Geometry: final body of the model. Coordinates: model frame, mm. A direction names the side the tool comes from. Give positions to 0.01 mm unless a question says otherwise; leave off trailing zeros. Loops run counter-clockwise (first coordinate to the right, second up) from the corner with the lowest first, then second, coordinate; pieces in that order, holes last. Notation, with made-up numbers: (21, -16.5) - (75, -16.5) arc R13 cw to (75, -2.5) - close; hole circle Ø5 at (-19, 72). An arc over 180 degrees is marked (long way). Answer in a Markdown table with one row per item.
from build123d import *

# Parameters (mm, degrees)
SKETCH1_W           = 406.4
SKETCH1_H           = 215.9
BOSS_EXTRUDE1_DEPTH = 12.7
SKETCH3_W           = 406.4
SKETCH3_H           = 190.5
CUT_EXTRUDE1_DEPTH  = 6.35


with BuildPart() as part:
    # Sketch1 → Boss-Extrude1 (new, symmetric)
    with BuildSketch(Plane.XY):
        Rectangle(SKETCH1_W, SKETCH1_H)
    extrude(amount=BOSS_EXTRUDE1_DEPTH, both=True)

    # Sketch3 → Cut-Extrude1 (cut)
    with BuildSketch(Plane.XY.offset(12.7)):
        with Locations((0, -12.7)):
            Rectangle(SKETCH3_W, SKETCH3_H)
    cut_extrude1 = extrude(amount=-CUT_EXTRUDE1_DEPTH, mode=Mode.SUBTRACT)

    # Mirror1: Cut-Extrude1 across plane
    add(cut_extrude1.mirror(Plane.XY), mode=Mode.SUBTRACT)


solid = part.part
Q1. Reachability of faces 1 (the flat face through (-3, -11, -6.35)), 2 (the flat face through (-3, -11, 6.35)), 3 (the flat face through (-3, 107.95, 0)) from +Z, -Z, +X, -X, +Y, -Y: full face, straight path, thin tool, end or side. Return the list, or none.
Check values:
| item | result |
|---|---|
| face 1 | -Z, +X, -X, -Y |
| face 2 | +Z, +X, -X, -Y |
| face 3 | +Z, -Z, +X, -X, +Y |
Q2. First-contact query: pin 1 (5 mm diameter, centred on x = 43, z = -9, fed in from -Y); pin 2 (1.5 mm diameter, centred on y = 53, z = 8.5, fed in from -X); pin 3 (4 mm diameter, centred on x = -45, y = -81, fed in from +Z). Flat tips, straight axial feed; report the tip coordinate or a pass-through.
Check values:
| item | result |
|---|---|
| pin 1 | y = 82.55 |
| pin 2 | through |
| pin 3 | z = 6.35 |
Q3. Cut plane B-B (y = -88.5). Output: boundary loops of the cut face in (x, z).
Check values:
| item | result |
|---|---|
| outline | (-203.2, -6.35) - (203.2, -6.35) - (203.2, 6.35) - (-203.2, 6.35) - close |
Q4. Material intervals for line 1 along Z through (x, y) = (20.5, -94.5); line 2 along Y through (x, z) = (-175.5, 9.5), sorted ascending.
Check values:
| item | result |
|---|---|
| line 1 | -6.35 to 6.35 |
| line 2 | 82.55 to 107.95 |
Q5. Cut plane A-A (x = -38). Output: boundary loops of the cut face in (y, z).
Check values:
| item | result |
|---|---|
| outline | (-107.95, -6.35) - (82.55, -6.35) - (82.55, -12.7) - (107.95, -12.7) - (107.95, 12.7) - (82.55, 12.7) - (82.55, 6.35) - (-107.95, 6.35) - close |
